Work out the finished part from the listing and answer in its coordinate system (mm). Give positions to 0.01 mm unless a question says otherwise; leave off trailing zeros. Write each loop counter-clockwise with the first axis right and the second up, starting at its lowest first coordinate (ties: lowest second). Pieces come first, ordered by that corner, then holes.
1) Straight lines are drawn through the part: probe 1 along Y at (x, z) = (-3, 0.5); probe 2 along Y at (x, z) = (-8, 2.55); probe 3 along X at (y, z) = (34, 1.95). For each, find the intervals that lie inside material, in ascending order.
2) Find section B-B (y = 0). Determine the outline of the cut face in (x, z) (3 decimals), plus the area to 4 significant figures.
3) Find section C-C (z = 2.1). Determine the outline of the cut face in (x, y).
4) Find section D-D (y = 44). Determine the outline of the cut face in (x, z) (3 decimals).
5) Find section A-A (x = 0). Determine the outline of the cut face in (y, z) (3 decimals).
6) Given pin 1 Ø6.5 at (x, y) = (0, 40) entering from -Z; pin 2 Ø1.6 at (y, z) = (39, 1) entering from -X, each flat-ended and moving along its own axis, determine where each tip first touches the part or whether it passes through.
```python
from build123d import *

# Parameters (mm, degrees)
ESBO_O1_R       = 5.25
EXTRUS_O1_DEPTH = 3.175
FILETE1_R       = 5


with BuildPart() as part:
    # Esboço1 → Extrusão1 (new body)
    with BuildSketch(Plane.XY):
        with BuildLine():
            ThreePointArc((-13.25, 32.664965942), (-32.643593337, 13.30256795), (-32.307158649, -14.1))
            Line((-32.307158649, -14.1), (-13.97685587, -56.1))
            ThreePointArc((-13.97685587, -56.1), (0, -65.25), (13.97685587, -56.1))
            Line((13.97685587, -56.1), (32.307158649, -14.1))
            ThreePointArc((32.307158649, -14.1), (32.643593337, 13.30256795), (13.25, 32.664965942))
            Line((13.25, 32.664965942), (13.25, 40))
            ThreePointArc((13.25, 40), (0, 53.25), (-13.25, 40))
            Line((-13.25, 40), (-13.25, 32.664965942))
        make_face()
        with Locations((0, 40)):
            Circle(ESBO_O1_R, mode=Mode.SUBTRACT)
        with Locations((0, -50)):
            Circle(ESBO_O1_R, mode=Mode.SUBTRACT)
        Circle(ESBO_O1_R, mode=Mode.SUBTRACT)
    extrude(amount=EXTRUS_O1_DEPTH)

    # Filete1
    filete1_edges = [part.edges().sort_by_distance(p)[0] for p in [
        (13.25, 32.664965942, 1.5875),
        (-13.25, 32.664965942, 1.5875),
    ]]
    fillet(filete1_edges, radius=FILETE1_R)


solid = part.part
```
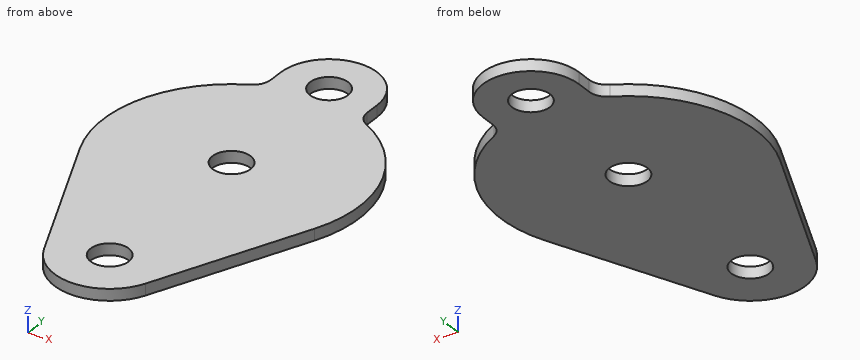
Results:
1. probe 1: y = -64.95 to -54.31, -45.69 to -4.31, 4.31 to 35.69, 44.31 to 52.91
1. probe 2: y = -62.98 to 50.56
1. probe 3: x = -13.61 to 13.61
2. outline: (-35.25, 0) - (-5.25, 0) - (-5.25, 3.175) - (-35.25, 3.175) - close; (5.25, 0) - (35.25, 0) - (35.25, 3.175) - (5.25, 3.175) - close
2. area: 190.5 mm2
3. outline: (-32.31, -14.1) - (-13.98, -56.1) arc R15.25 ccw to (13.98, -56.1) - (32.31, -14.1) arc R35.25 ccw to (15.98, 31.42) arc R5 cw to (13.25, 35.87) - (13.25, 40) arc R13.25 ccw to (-13.25, 40) - (-13.25, 35.87) arc R5 cw to (-15.98, 31.42) arc R35.25 ccw to start; hole circle Ø10.5 at (0, -50); hole circle Ø10.5 at (0, 0); hole circle Ø10.5 at (0, 40)
4. outline: (-12.632, 0) - (-3.4, 0) - (-3.4, 3.175) - (-12.632, 3.175) - close; (3.4, 0) - (12.632, 0) - (12.632, 3.175) - (3.4, 3.175) - close
5. outline: (-65.25, 0) - (-55.25, 0) - (-55.25, 3.175) - (-65.25, 3.175) - close; (-44.75, 0) - (-5.25, 0) - (-5.25, 3.175) - (-44.75, 3.175) - close; (5.25, 0) - (34.75, 0) - (34.75, 3.175) - (5.25, 3.175) - close; (45.25, 0) - (53.25, 0) - (53.25, 3.175) - (45.25, 3.175) - close
6. pin 1: passes through
6. pin 2: stops at x = -13.25
